Read the model definition and answer for the solid it produces. Units are mm, in the model's axes. A direction names the side the tool comes from. Round coordinates to 2 decimals unless told otherwise and drop trailing zeros. Write each loop counter-clockwise with the first axis right and the second up, starting at its lowest first coordinate (ties: lowest second). Pieces come first, ordered by that corner, then holes. Notation, with made-up numbers: (48, 51.25) - (61, 51.25) arc R29 ccw to (61, 84.25) - close; hole circle Ø9 at (23.25, -35.5). An arc over 180 degrees is marked (long way). Use one line per item in the form item = value. Start each with the question number.
1) For faces 1 (the face through (-2.193, 49, 8)), 2 (the face through (26, 49, 44.25)), determine the directions among +Z, -Z, +X, -X, +Y, -Y from which every point of the face is accessible in a straight line to the end or side of a thin tool.
2) The part is cut by section B-B, the plane y = 57. Give the vertices of the cut face in (x, z), plus the area to 3 significant figures.
3) The part is cut by section C-C, the plane z = -19.5. Give the vertices of the cut face in (x, y), plus the area to 3 significant figures.
4) Each of these flat-tipped pins is pushed along its axis until it touches: pin 1 (4 mm diameter, centred on x = 38.5, y = 22.5, fed in from -Z); pin 2 (4 mm diameter, centred on y = 79, z = -13, fed in from +X); pin 3 (4 mm diameter, centred on y = 84, z = -31, fed in from +X); pin 4 (12 mm diameter, centred on x = 41, z = -86, fed in from +Y). Where does it stop, or does it pass through?
5) The part is cut by section A-A, the plane x = 15. Give the vertices of the cut face in (y, z).
6) Consider line 1 along Z through (x, y) = (33.5, 30); line 2 along Z through (x, y) = (46, 46); line 3 along X through (y, z) = (24, 7). Determine where each line is inside the solid, lowest interval first. Write a range as from..to.
from build123d import *

# Parameters (mm, degrees)
BOSS_EXTRUDE1_DEPTH = 100
SKETCH2_W           = 3.749917695
SKETCH2_H           = 0.25242756
SKETCH2_H_2         = 0.267899142
SKETCH2_H_3         = 0.289005846
SKETCH2_H_4         = 0.253626666
SKETCH2_H_5         = 0.325456574
SKETCH2_H_6         = 0.248885072
SKETCH2_H_7         = 0.22456854
SKETCH2_H_8         = 0.302440332
SKETCH2_H_9         = 0.27412506
CUT_EXTRUDE1_DEPTH  = 1
SKETCH3_W           = 0.401370442
SKETCH3_H           = 3.749917695
SKETCH3_W_2         = 0.402319906
SKETCH3_W_3         = 0.403269369
SKETCH3_W_4         = 0.379270676
CUT_EXTRUDE2_DEPTH  = 1


with BuildPart() as part:
    # Sketch1 → Boss-Extrude1 (new body)
    with BuildSketch(Plane(origin=(0, 0, 0), x_dir=(1, 0, 0), z_dir=(0, 1, 0))):
        Polygon((0.807035346, 30), (50.807035346, 116.602540378), (48.557035346, 117.901578484), (-2.192964654, 30), (-2.192964654, 0), (-2.192964654, -48), (50.807035346, -48), (50.807035346, -44.250082305), (0.807035346, -44.250082305), (0.807035346, -10), (0.807035346, 3.423298646), align=None)
    extrude(amount=BOSS_EXTRUDE1_DEPTH)

    # Sketch2 → Cut-Extrude1 (cut)
    with BuildSketch(Plane(origin=(50.807035346, 0, 0), x_dir=(0, 0, -1), z_dir=(1, 0, 0))):
        with Locations((-46.125041153, 90)):
            Rectangle(SKETCH2_W, SKETCH2_H)
        with Locations((-46.125041153, 80)):
            Rectangle(SKETCH2_W, SKETCH2_H_2)
        with Locations((-46.125041153, 70)):
            Rectangle(SKETCH2_W, SKETCH2_H_3)
        with Locations((-46.125041153, 60)):
            Rectangle(SKETCH2_W, SKETCH2_H_4)
        with Locations((-46.125041153, 50)):
            Rectangle(SKETCH2_W, SKETCH2_H_5)
        with Locations((-46.125041153, 40)):
            Rectangle(SKETCH2_W, SKETCH2_H_6)
        with Locations((-46.125041153, 30)):
            Rectangle(SKETCH2_W, SKETCH2_H_7)
        with Locations((-46.125041153, 20)):
            Rectangle(SKETCH2_W, SKETCH2_H_8)
        with Locations((-46.125041153, 10)):
            Rectangle(SKETCH2_W, SKETCH2_H_9)
    extrude(amount=-CUT_EXTRUDE1_DEPTH, mode=Mode.SUBTRACT)

    # Sketch3 → Cut-Extrude2 (cut)
    with BuildSketch(Plane(origin=(0, 100, 0), x_dir=(1, 0, 0), z_dir=(0, 1, 0))):
        with Locations((40.807035346, -46.125041153)):
            Rectangle(SKETCH3_W, SKETCH3_H)
        with Locations((30.807035346, -46.125041153)):
            Rectangle(SKETCH3_W_2, SKETCH3_H)
        with Locations((20.807035346, -46.125041153)):
            Rectangle(SKETCH3_W_3, SKETCH3_H)
        with Locations((10.807035346, -46.125041153)):
            Rectangle(SKETCH3_W_4, SKETCH3_H)
    extrude(amount=-CUT_EXTRUDE2_DEPTH, mode=Mode.SUBTRACT)


solid = part.part
Geometry results:
q1.face_1 = +Z, -Z, -X, +Y, -Y
q1.face_2 = +X, +Y, -Y
q2.outline = (-2.19, -30) - (48.56, -117.9) - (50.81, -116.6) - (0.81, -30) - (0.81, 44.25) - (50.81, 44.25) - (50.81, 48) - (-2.19, 48) - close
q2.area = 683 mm2
q3.outline = (-2.19, 0) - (0.81, 0) - (0.81, 100) - (-2.19, 100) - close
q3.area = 300 mm2
q4.pin_1 = -103.95
q4.pin_2 = 0.81
q4.pin_3 = 2.54
q4.pin_4 = through
q5.outline = (0, -59.78) - (100, -59.78) - (100, -54.58) - (0, -54.58) - close; (0, 44.25) - (100, 44.25) - (100, 48) - (0, 48) - close
q6.line_1 = -91.82..-86.63, 44.25..48
q6.line_2 = -113.47..-108.28, 44.25..48
q6.line_3 = -2.19..0.81
